Verification items for this drawing (mm, ordinates from the low corner). A direction names the side the tool comes from. Round coordinates to 2 decimals unless told otherwise and drop trailing zeros. Order: outer loops, then holes, each group sorted by start corner. A loop starts at its lowest first (then second) coordinate and runs counter-clockwise, first axis right, second up. Notation, with made-up numbers: (-5, 27) -> (51, 27) arc R21 ccw to (51, 52) -> close; hole circle Ø5 at (20.5, -32). An arc over 180 degrees is marked (long way). Answer in a Markdown table with one row per item. Add a question column.
1. Draft check along Y on the marked faces 1, 2 and 3. Enter one of: +Y half, -Y half, draft (parallel to the pull), parting line (faces both ways), or undercut.
2. Material ranges on L1, parallel to Y at x = 6.25, z = 5.5; L2, parallel to Y at x = 3.25, z = 1.5; L3, parallel to Z at x = 4, y = 10, recorded low to high. Write a range as from..to.
3. Access from +Z, -Z, +X, -X, +Y, -Y to the whole of each face (thin tool, end or side, straight path). Record for the marked faces 4, 5, 6, 7 and 8.
4. Sectioned sample at C-C, the plane x = 6.5. Record the boundary of the cut face in (y, z).
5. Sectioned sample at B-B, the plane y = 5.5. Record the boundary of the cut face in (x, z).
6. Sectioned sample at A-A, the plane z = 5. Record the boundary of the cut face in (x, y).
7. Sectioned sample at D-D, the plane z = 1. Record the boundary of the cut face in (x, y).
8. Depth check by flat-ended pin: P1, Ø2.5, axis at x = 5, y = 18.5, coming from the -Z side; P2, Ø1.5, axis at y = 3.5, z = 1.5, coming from the -X side. Enter the tip coordinate at first touch or a pass-through.
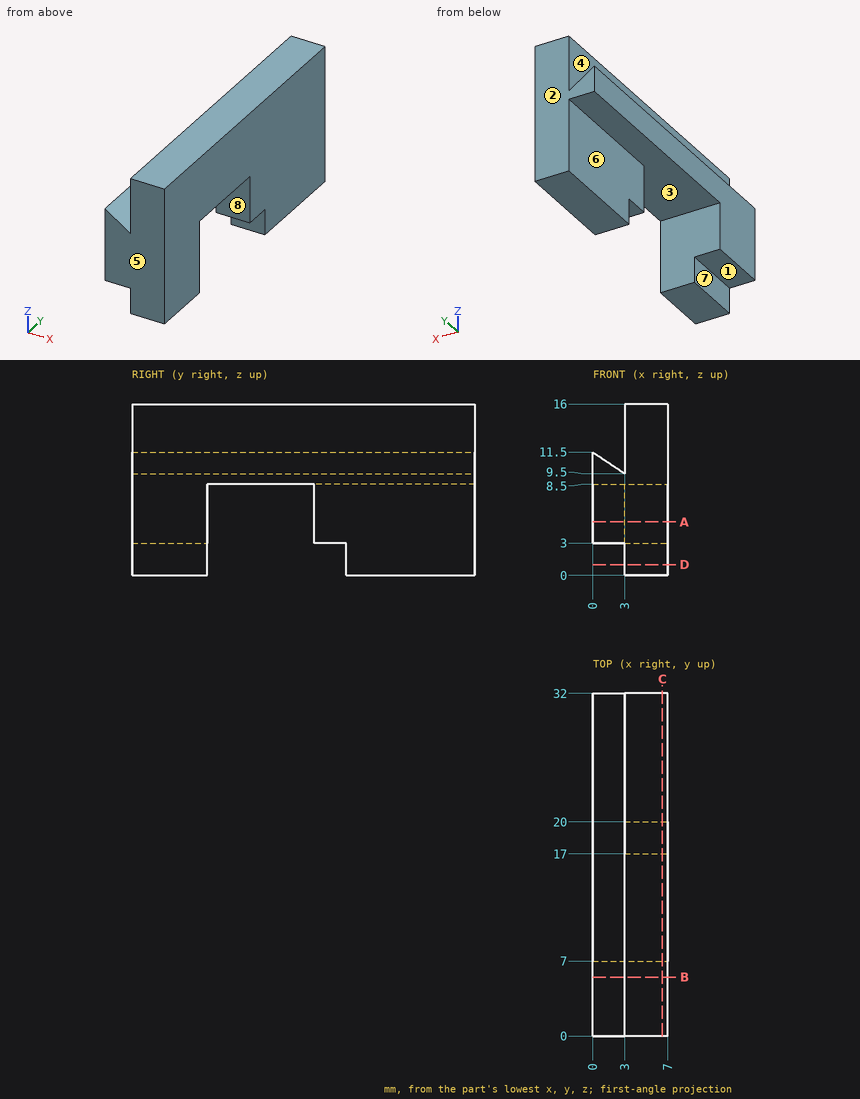
Answer key:
| question | item | result |
|---|---|---|
| 1 | face 1 | draft |
| 1 | face 2 | +Y half |
| 1 | face 3 | undercut |
| 2 | L1 | y = 0..7, 17..32 |
| 2 | L2 | y = 0..7, 20..32 |
| 2 | L3 | z = 8.5..16 |
| 3 | face 4 | +Z, +Y, -Y |
| 3 | face 5 | +Z, -Z, +X, -X, -Y |
| 3 | face 6 | -Z, -X, +Y |
| 3 | face 7 | -Z, -X, +Y, -Y |
| 3 | face 8 | -Z, +X, -X |
| 4 | outline | (0, 0) -> (7, 0) -> (7, 8.5) -> (17, 8.5) -> (17, 3) -> (20, 3) -> (20, 0) -> (32, 0) -> (32, 16) -> (0, 16) -> close |
| 5 | outline | (0, 3) -> (3, 3) -> (3, 0) -> (7, 0) -> (7, 16) -> (3, 16) -> (3, 9.5) -> (0, 11.5) -> close |
| 6 | outline | (0, 0) -> (7, 0) -> (7, 7) -> (0, 7) -> close; (3, 17) -> (7, 17) -> (7, 32) -> (3, 32) -> close |
| 7 | outline | (3, 0) -> (7, 0) -> (7, 7) -> (3, 7) -> close; (3, 20) -> (7, 20) -> (7, 32) -> (3, 32) -> close |
| 8 | P1 | stops at z = 3 |
| 8 | P2 | stops at x = 3 |
